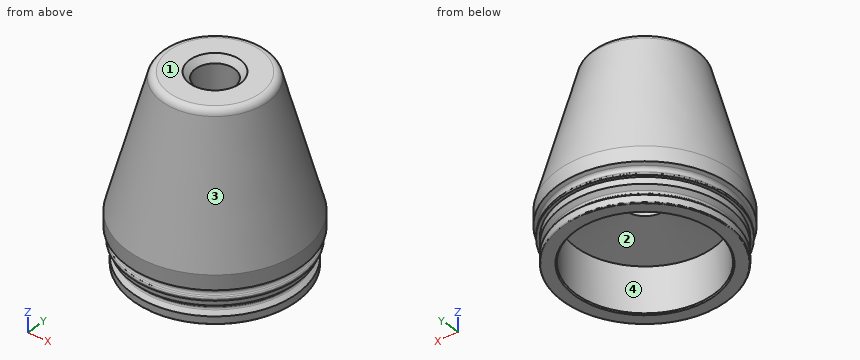
```python
from build123d import *


with BuildPart() as part:
    # Sketch3 → FBR-00 Basic blank revolve (revolve)
    with BuildSketch(Plane(origin=(0, 0, 0), x_dir=(0, 0, -1), z_dir=(1, 0, 0)), mode=Mode.PRIVATE) as fbr_00_basic_blank_revolve_sk:
        with BuildLine():
            Line((-53.109996064, 18.328023479), (-9.057762175, 30.1625))
            Line((-9.057762175, 30.1625), (-3.977762175, 30.1625))
            Line((-3.977762175, 30.1625), (-3.385852263, 29.137281959))
            ThreePointArc((-3.385852263, 29.137281959), (-2.451768264, 28.513146985), (-1.387974388, 28.874256347))
            Line((-1.387974388, 28.874256347), (-1.046815367, 29.215415367))
            ThreePointArc((-1.046815367, 29.215415367), (-0.799604775, 29.380596204), (-0.508, 29.4386))
            Line((-0.508, 29.4386), (0, 29.4386))
            Line((0, 29.4386), (0, 28.448))
            Line((0, 28.448), (2.260600025, 28.448))
            Line((2.260600025, 28.448), (3.525184633, 27.183415393))
            ThreePointArc((3.525184633, 27.183415393), (4.064, 26.96023076), (4.602815367, 27.183415393))
            Line((4.602815367, 27.183415393), (5.867399975, 28.448))
            Line((5.867399975, 28.448), (8.255, 28.448))
            ThreePointArc((8.255, 28.448), (8.434605122, 28.373605122), (8.509, 28.194))
            Line((8.509, 28.194), (8.509, 24.1935))
            Line((8.509, 24.1935), (8.128, 23.8125))
            Line((8.128, 23.8125), (-7.366, 23.8125))
            Line((-7.366, 23.8125), (-11.939571176, 6.7437))
            Line((-11.939571176, 6.7437), (-52.959, 6.7437))
            Line((-52.959, 6.7437), (-54.991, 8.7757))
            Line((-54.991, 8.7757), (-54.991, 15.875))
            ThreePointArc((-54.991, 15.875), (-54.466620252, 17.420598589), (-53.109996064, 18.328023479))
        make_face()
    revolve(fbr_00_basic_blank_revolve_sk.sketch.rotate(Axis((0, 0, 47.572309729), (0, 0, 1)), 90), axis=Axis((0, 0, 47.572309729), (0, 0, 1)))


solid = part.part
```
Design review of the part built by this model. Coordinates are the model's own, in mm. Face numbers are marked on the shaded views. Round coordinates to 2 decimals unless told otherwise and drop trailing zeros. Order: outer loops, then holes, each group sorted by start corner. A loop starts at its lowest first (then second) coordinate and runs counter-clockwise, first axis right, second up. Notation, with made-up numbers: (54, 3.5) - (85, 3.5) arc R15 cw to (85, 9.5) - close; hole circle Ø10 at (56, 20.5). An arc over 180 degrees is marked (long way). Return JSON: item names as keys, results as strings.
Q1. The part is to be moulded in two halves that separate along Y. For the marked faces 1, 2, 3 and 4, say which applies: pulls with the +Y half, pulls with the -Y half, needs draft (parallel to the pull), parting line crosses it, or undercut.
Computed values:
{"face 1": "needs draft", "face 2": "undercut", "face 3": "parting line crosses it", "face 4": "undercut"}
Q2. Consider section B-B on z = 50. Write out the cut boundary in (x, y), plus the area to 3 significant figures.
Computed values:
{"outline": "circle Ø38.33 at (0, 0); hole circle Ø13.49 at (0, 0)", "area": "1,010 mm2"}
Q3. Wall thickness on L1, parallel to X at y = -1.5, z = 26; L2, parallel to Y at x = -13.5, z = -3.5; L3, parallel to Y at x = -14.5, z = -3: over which ranges is each line inside the solid? List them lowest first. Write a range as [from, to].
Computed values:
{"L1": "x = [-25.57, -6.57], [6.57, 25.57]", "L2": "y = [-23.62, -19.62], [19.62, 23.62]", "L3": "y = [-23.61, -18.89], [18.89, 23.61]"}
Q4. Consider section A-A on z = 35. Write out the cut boundary in (x, y).
Computed values:
{"outline": "circle Ø46.39 at (0, 0); hole circle Ø13.49 at (0, 0)"}
Q5. For pin 1 Ø8 at (x, z) = (-11, 39) entering from +Y; pin 2 Ø17.5 at (x, y) = (0, 0) entering from -Z; pin 3 Ø2 at (x, z) = (-5.5, 39.5) entering from +Y, all flat-tipped, find the tip position at first contact; note any pin that passes through.
Computed values:
{"pin 1": "stops at y = 21.39", "pin 2": "stops at z = 11.4", "pin 3": "stops at y = 21.65"}
